Autodesk Inventor part; units mm, degrees
ref_plane "YZ Plane" through (0, 0, 0) normal (1, 0, 0) x (0, 1, 0)
ref_plane "XZ Plane" through (0, 0, 0) normal (0, 1, 0) x (-1, 0, 0)
ref_plane "XY Plane" through (0, 0, 0) normal (0, 0, 1) x (1, 0, 0)
sketch "Boceto1" plane through (0, 0, 0) normal (0, 0, 1) x (1, 0, 0)
  line L0 (0, 0) -> (487.58, 0)
  line L1 (487.58, 0) -> (487.58, 337.58)
  line L2 (487.58, 337.58) -> (0, 337.58)
  line L3 (0, 337.58) -> (0, 0)
  dimension "d0" = 487.58
  dimension "d1" = 337.58
extrude "Placa1" add sketch "Boceto1" along normal blind 0.76
sketch "Boceto2" plane through (487.58, 0.76, 0) normal (0, -1, 0) x (1, 0, 0)
  line L0 (-487.58, 0) -> (0, 0)
  line L1 (0, 0) -> (0, 25)
  line L2 (0, 25) -> (-487.58, 25)
  line L3 (-487.58, 25) -> (-487.58, 0)
edge flange "Pestaña1" height 25 angle 90 thickness 0.76 bend radius 0.76 thickness toward (0, -1, 0) relief tear relief width 0.76 relief depth 0.38 edges at (243.79, 0, 0.76) wall of the first edge with corners at (0, 0.76, 0) (487.58, 0.76, 0) (487.58, 0.76, 25) (0, 0.76, 25)
bend "Doblez1"
corner "Esquina1"
sketch "Boceto3" plane through (0, 0, 0) normal (0, 0, -1) x (-1, 0, 0)
  circle A0 centre (-469.48, 308.225) radius 2.5
  circle A1 centre (-243.79, 308.225) radius 2.5
  circle A2 centre (-18.1, 308.225) radius 2.5
  point P0 (0, 0)
extrude "Cortar1" cut sketch "Boceto3" against normal blind 0.76
sketch "Boceto4" plane through (0, 0.76, 25) normal (0, 1, 0) x (1, 0, 0)
  line L0 (0, 23.48) -> (0, 0)
  line L1 (487.58, 23.48) -> (487.58, 0)
  line L2 (0, 0) -> (487.58, 0)
  line L3 (0, 23.48) -> (487.58, 23.48)
  line L4 (0, 23.48) -> (0, 0)
  circle A0 centre (60, 11.74) radius 2.5
  circle A1 centre (243.79, 11.74) radius 2.5
  circle A2 centre (427.58, 11.74) radius 2.5
  point P0 (0, 25)
  dimension "d15" = 60
  dimension "d16" = 60
  dimension "d17" = 5
  dimension "d18" = 5
  dimension "d19" = 5
extrude "Extrusión1" cut sketch "Boceto4" against normal through all contours A0 | A1 | A2
thread "Rosca1"
thread "Rosca2"
thread "Rosca3"
equation "\"d13\" = Grosor"
equation "\"d18\" = d17"
equation "\"d19\" = d17"
equation "\"d2\" = Grosor"
equation "\"d3\" = Anchura_desahogo_plegado"
equation "\"d4\" = Profundidad_desahogo_plegado"
equation "\"d5\" = Remanente_mínimo"
equation "\"d6\" = Radiodetransición"
equation "\"d9\" = Radio_pliegue"
equation "\"d10\" = Tamaño_destalonado"
equation "\"d11\" = TamañoSeparación"
equation "\"d12\" = Tamaño_de_radio_de_Jacobi"
equation "\"Radio_pliegue\" = Grosor"
equation "\"Anchura_desahogo_plegado\" = Grosor"
equation "\"Profundidad_desahogo_plegado\" = 0.5 * Grosor"
equation "\"Tamaño_destalonado\" = 4 * Grosor"
equation "\"Remanente_mínimo\" = 2 * Grosor"
equation "\"Radiodetransición\" = Radio_pliegue"
equation "\"Tamaño_de_radio_de_Jacobi\" = Radio_pliegue"
equation "\"TamañoSeparación\" = Grosor"
properties part number "Tapa_interior_2" material "Acero AISI 1006 85 LC"
Source: CAD feature listing. Evaluate the final solid. Frame: model axes, mm. A direction names the side the tool comes from. Coordinates: 2 decimals unless noted, no trailing zeros. Write each loop counter-clockwise with the first axis right and the second up, starting at its lowest first coordinate (ties: lowest second). Pieces come first, ordered by that corner, then holes. Notation, with made-up numbers: (52, 24) -> (76, 24) arc R13 ccw to (76, 48) -> close; hole circle Ø4 at (75, 12.25). An arc over 180 degrees is marked (long way). Return JSON: item names as keys, results as strings. Group by question number.
1) Contact query for flat-ended pins moving along their axis: P1, Ø1.5, axis at x = 186.5, z = 14, coming from the -Y side; P2, Ø4.5, axis at x = 427.58, z = 13.26, coming from the +Y side; P3, Ø11.5, axis at x = 333, z = 15, coming from the +Y side; P4, Ø2, axis at x = 302, y = 63.5, coming from the +Z side. Output: stop coordinate, or through.
2) Set-up query: faces 1 (the face through (247, 0.76, 13)), 2 (the face through (240, 172, 0)). Return all of +Z, -Z, +X, -X, +Y, -Y with unobstructed straight access to the full face (end or side cutting, diameter ignored); none if empty.
3) Section query A-A, the plane x = 85. Return loops of the section in (y, z).
4) Section query B-B, the plane y = 193. Return loops of the section in (x, z), plus the area to 3 significant figures.
5) Ray query, line 1 along X through (y, z) = (0.35, 13.26); line 2 along Y through (x, z) = (21.5, 4). Return the intervals inside material, ascending.
From the geometry:
{
 "1": {"P1": "y = 0", "P2": "through", "P3": "y = 0.76", "P4": "z = 0.76"},
 "2": {"face 1": "+Z, +X, -X, +Y", "face 2": "-Z, +X, -X, +Y, -Y"},
 "3": {"outline": "(0, 1.52) arc R1.52 ccw to (1.52, 0) -> (337.58, 0) -> (337.58, 0.76) -> (1.52, 0.76) arc R0.76 cw to (0.76, 1.52) -> (0.76, 25) -> (0, 25) -> close"},
 "4": {"outline": "(0, 0) -> (487.58, 0) -> (487.58, 0.76) -> (0, 0.76) -> close", "area": "371 mm²"},
 "5": {"line 1": "0 to 57.5, 62.5 to 241.29, 246.29 to 425.08, 430.08 to 487.58", "line 2": "0 to 0.76"}
}
